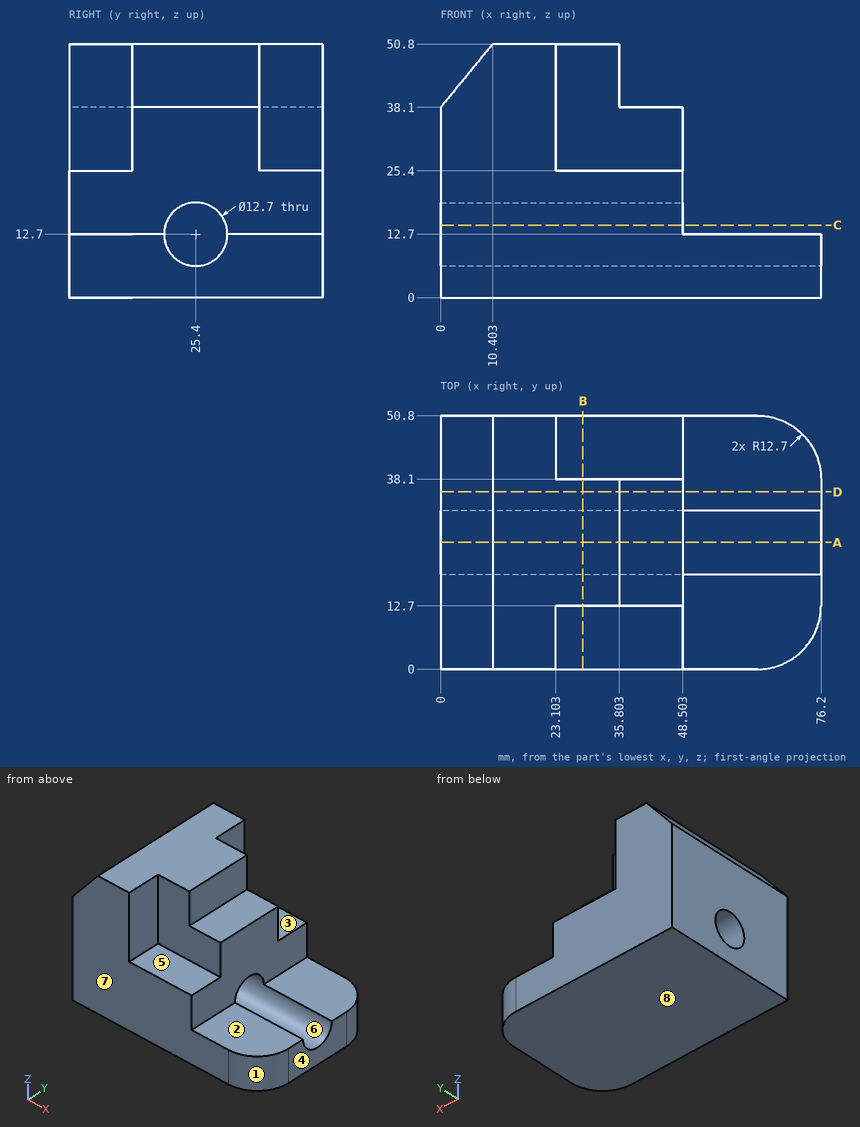
Answer from the drawing. Dimensions are ordinates in mm from the lowest x, y and z of the part. A direction names the side the tool comes from. Give positions to 0.01 mm unless a question says otherwise; leave off trailing zeros. Write each loop counter-clockwise with the first axis right and the second up, starting at its lowest first coordinate (ties: lowest second). Pieces come first, ordered by that corner, then holes. Notation, with made-up numbers: M 62,34 L 91,34 A18 cw 91,53 Z; hole C -36.5,-22.5 d5. An arc over 180 degrees is marked long. Answer as CSV lines item,"result".
Q1. A cutting plane is placed at B-B on x = 28.5. Write down the section's boundary in (y, z).
A:
outline,"M 0,0 L 50.8,0 L 50.8,25.4 L 38.1,25.4 L 38.1,50.8 L 12.7,50.8 L 12.7,25.4 L 0,25.4 Z; hole C 25.4,12.7 d12.7"
Q2. A cutting plane is placed at D-D on y = 35.5. Write down the section's boundary in (x, z).
A:
outline,"M 0,0 L 76.2,0 L 76.2,12.7 L 48.5,12.7 L 48.5,38.1 L 35.8,38.1 L 35.8,50.8 L 10.4,50.8 L 0,38.1 Z"
Q3. The mould has two halves that part along Y. Classify the marked faces 6, 7 and 8: +Y half, -Y half, draft (parallel to the pull), parting line (faces both ways), or undercut.
A:
face 6,"undercut"
face 7,"-Y half"
face 8,"draft"
Q4. A tool of negligible diameter and unlimited length cuts with its end or side. For the marked faces 1, 2, 3, 4 and 5, from which of +Z, -Z, +X, -X, +Y, -Y can it reach the whole face along a straight path? Write none if from no direction.
A:
face 1,"+Z, -Z, +X, -Y"
face 2,"+Z, +X, +Y, -Y"
face 3,"+Z, +X, +Y"
face 4,"+Z, -Z, +X, +Y, -Y"
face 5,"+Z, +X, -Y"
Q5. Find the intervals of material crossed by probe 1 along Z at (x, y) = (46, 25.4); probe 2 along Y at (x, z) = (42.5, 12.7); probe 3 along Z at (x, y) = (31.5, 25.4), in increasing order. Write a range as [from, to].
A:
probe 1,"z = [0, 6.35], [19.05, 38.1]"
probe 2,"y = [0, 19.05], [31.75, 50.8]"
probe 3,"z = [0, 6.35], [19.05, 50.8]"
Q6. Given P1, Ø14, axis at x = 36.5, y = 47.5, coming from the +Z side; P2, Ø7.5, axis at y = 13.5, z = 20, coming from the +X side; P3, Ø4, axis at y = 5, z = 39.5, coming from the +X side; P4, Ø10, axis at x = 32, y = 39, coming from the -Z side, each flat-ended and moving along its own axis, determine where each tip first touches the part or whether it passes through.
A:
P1,"stops at z = 25.4"
P2,"stops at x = 48.5"
P3,"stops at x = 23.1"
P4,"stops at z = 0"
Q7. A cutting plane is placed at A-A on y = 25.4. Write down the section's boundary in (x, z), plus the area to 3 significant figures.
A:
outline,"M 0,0 L 76.2,0 L 76.2,6.35 L 0,6.35 Z; M 0,19.05 L 48.5,19.05 L 48.5,38.1 L 35.8,38.1 L 35.8,50.8 L 10.4,50.8 L 0,38.1 Z"
area,"1,800 mm²"
Q8. A cutting plane is placed at C-C on z = 14.5. Write down the section's boundary in (x, y).
A:
outline,"M 0,0 L 48.5,0 L 48.5,19.31 L 0,19.31 Z; M 0,31.49 L 48.5,31.49 L 48.5,50.8 L 0,50.8 Z"
